Source: three-view drawing plus pictorial views. Frame: mm from the lowest corner of the part. A direction names the side the tool comes from. Give positions to 0.01 mm unless a question says otherwise; leave off trailing zeros. Loops run counter-clockwise (first coordinate to the right, second up) from the corner with the lowest first, then second, coordinate; pieces in that order, holes last.
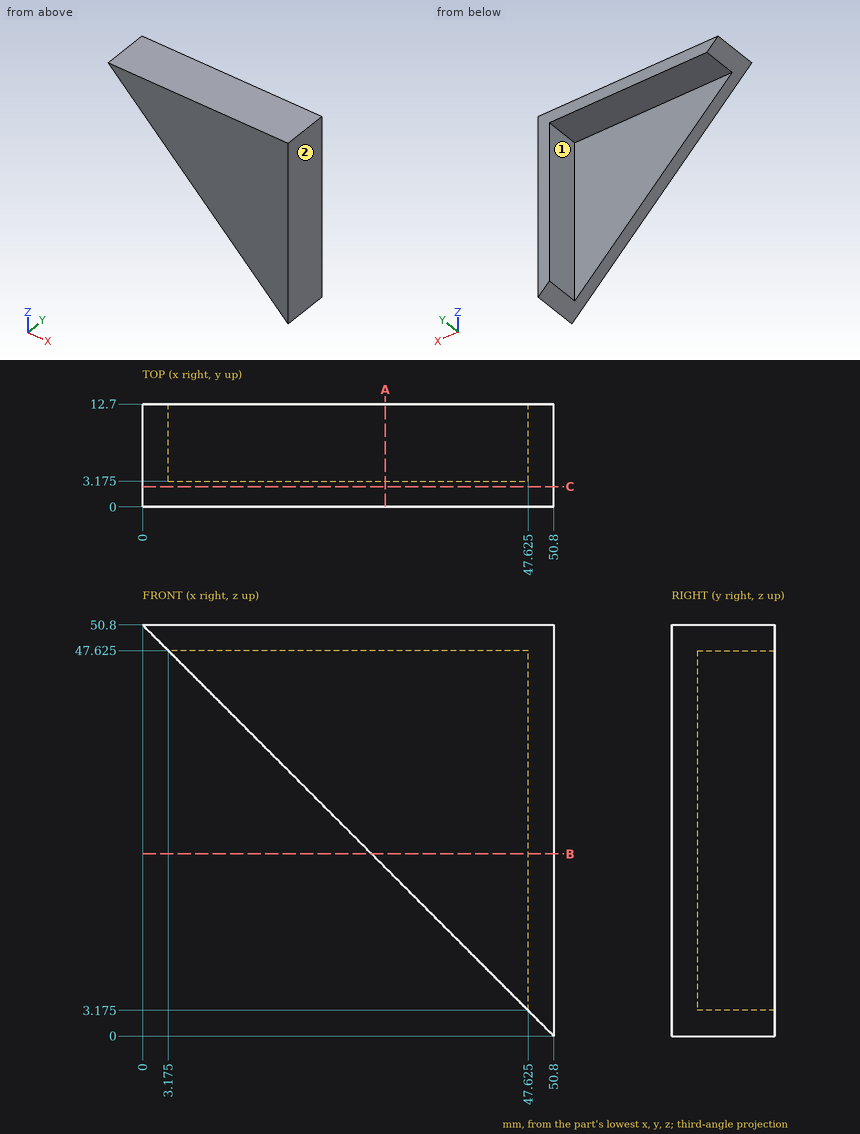
1) Ray query, probe 1 along Z at (x, y) = (4, 6) (3 decimals); probe 2 along Y at (x, z) = (27, 29) (3 decimals). Return the intervals inside material, ascending.
Checks:
probe 1: z = 47.625 to 50.8
probe 2: y = 0 to 3.175
2) Reachability of the marked faces 1 and 2 from +Z, -Z, +X, -X, +Y, -Y: full face, straight path, thin tool, end or side. Return the list, or none.
Checks:
face 1: -Z, -X, +Y
face 2: +Z, -Z, +X, +Y, -Y
3) Cut plane B-B (z = 22.5). Return loops of the section in (x, y) (3 decimals), and give its area (3 significant figures).
Checks:
outline: (28.3, 0) - (50.8, 0) - (50.8, 12.7) - (47.625, 12.7) - (47.625, 3.175) - (28.3, 3.175) - close
area: 102 mm2
4) Cut plane A-A (x = 30). Return loops of the section in (y, z) (3 decimals), and give its area (3 significant figures).
Checks:
outline: (0, 20.8) - (3.175, 20.8) - (3.175, 47.625) - (12.7, 47.625) - (12.7, 50.8) - (0, 50.8) - close
area: 125 mm2
5) Contact query for flat-ended pins moving along their axis: P1, Ø3, axis at y = 2, z = 8, coming from the -X side; P2, Ø5, axis at x = 38, z = 36, coming from the -Y side; P3, Ø22, axis at x = 16, z = 26, coming from the +Y side (3 decimals); P4, Ø3, axis at y = 8, z = 28, coming from the -X side (3 decimals). Output: stop coordinate, or through.
Checks:
P1: stops at x = 41.3
P2: stops at y = 0
P3: stops at y = 3.175
P4: stops at x = 47.625
6) Cut plane C-C (y = 2.5). Return loops of the section in (x, z), and give its area (3 significant figures).
Checks:
outline: (0, 50.8) - (50.8, 0) - (50.8, 50.8) - close
area: 1,290 mm2
